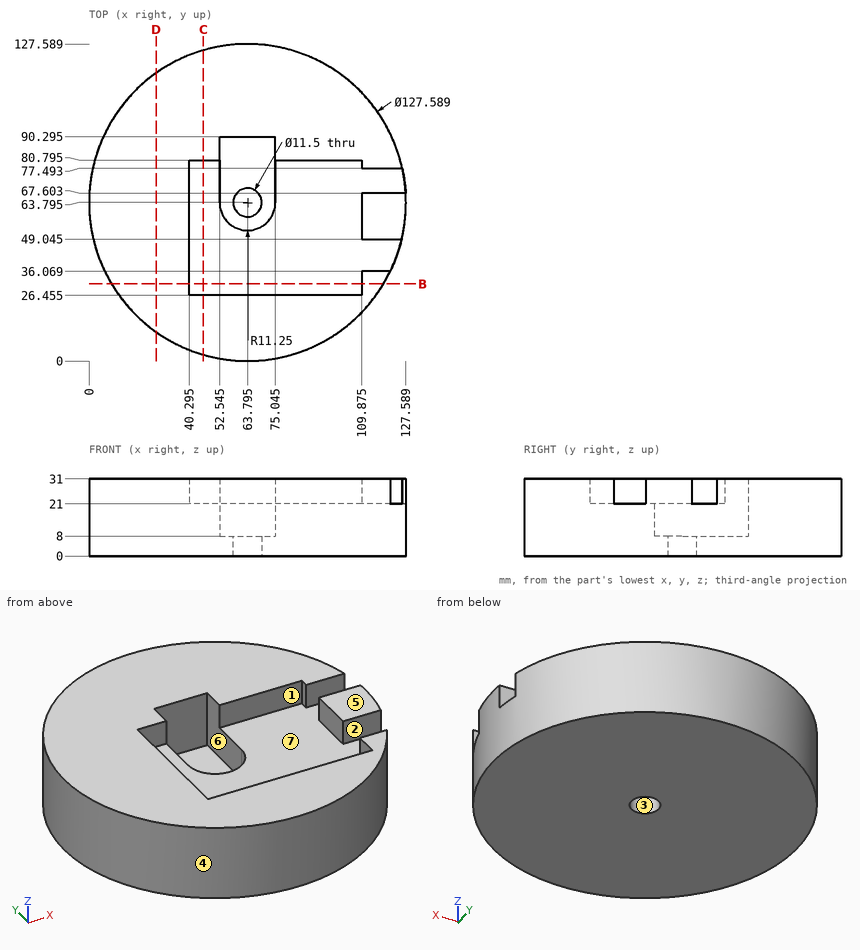
Can you work these out from the drawing? Everything is in mm from the part's minimum corner. A direction names the side the tool comes from. Coordinates: 2 decimals unless noted, no trailing zeros. Order: outer loops, then holes, each group sorted by start corner. A loop starts at its lowest first (then second) coordinate and runs counter-clockwise, first axis right, second up. Notation, with made-up numbers: M 54,-34.5 L 82,-34.5 A18 cw 82,-3.5 Z; hole C -21.75,64 d7. An arc over 180 degrees is marked long. Answer as CSV lines item,"result". Start each with the question number.
1. I want a section at B-B, the plane y = 31. Write out the boundary of the cut face in (x, z) (1 decimal).
2. On a 3-axis mill with a long thin cutter (end or side, diameter ignored), from which of +Z, -Z, +X, -X, +Y, -Y can I reach the whole of each face in a straight line? I mean the marked faces 1, 2 and 3. Say none if no direction works.
3. I need wall thicknesses on line 1 (Z direction, x = 93, y = 33); line 2 (Y direction, x = 73.5, z = 29) (1 decimal); line 3 (X direction, y = 85.5, z = 20) (1 decimal). Which ranges of each line are inside material? Lowest first, please. Write a range as [from, to].
4. For pin 1 (11 mm diameter, centred on x = 118, z = 28, fed in from -Y) (1 decimal); pin 2 (1 mm diameter, centred on y = 59.5, z = 22.5, fed in from +X); pin 3 (5 mm diameter, centred on y = 74, z = 12, fed in from +X), each with a flat end and sliding along its axis, tell me the tip position at first contact or that it passes through.
5. I want a section at C-C, the plane x = 46. Write out the boundary of the cut face in (y, z) (1 decimal), and give its area (4 significant figures).
6. We'd pull the mould along Y, two halves only. Please class the marked faces 4, 5, 6 and 7: released by +Y, released by -Y, zero draft, split by the parting line, or undercut.
7. I want a section at D-D, the plane x = 27. Write out the boundary of the cut face in (y, z).
Recorded:
1,outline,"M 9.1,0 L 118.5,0 L 118.5,31 L 109.9,31 L 109.9,21 L 40.3,21 L 40.3,31 L 9.1,31 Z"
2,face 1,"+Z"
2,face 2,"+Z, +X"
2,face 3,"+Z, -Z"
3,line 1,"z = [0, 21]"
3,line 2,"y = [0.7, 26.5], [90.3, 126.8]"
3,line 3,"x = [3.8, 52.5], [75, 123.8]"
4,pin 1,"stops at y = 22.6"
4,pin 2,"stops at x = 127.48"
4,pin 3,"stops at x = 127.12"
5,outline,"M 2.5,0 L 125.1,0 L 125.1,31 L 80.8,31 L 80.8,21 L 26.5,21 L 26.5,31 L 2.5,31 Z"
5,area,"3,255 mm2"
6,face 4,"split by the parting line"
6,face 5,"zero draft"
6,face 6,"undercut"
6,face 7,"undercut"
7,outline,"M 11.68,0 L 115.91,0 L 115.91,31 L 11.68,31 Z"
